```python
from build123d import *

# Parameters (mm, degrees)
SCHIZZO1_W                   = 22
SCHIZZO1_H                   = 10.6
ESTRUSIONE_ESTRUSIONE1_DEPTH = 15
TAGLIO_ESTRUSIONE3_REACH     = 23.409
SCHIZZO5_R                   = 1.75
SCHIZZO5_3_W                 = 6.5
SCHIZZO5_3_H                 = 30
TAGLIO_ESTRUSIONE4_DEPTH     = 0.6


with BuildPart() as part:
    # Schizzo1 → Estrusione-Estrusione1 (new, symmetric)
    with BuildSketch(Plane.XY):
        Rectangle(SCHIZZO1_W, SCHIZZO1_H)
    extrude(amount=ESTRUSIONE_ESTRUSIONE1_DEPTH, both=True)

    # Schizzo5 → Taglio-Estrusione3 (cut, up to next)
    with BuildSketch(Plane(origin=(0, 5.3, 0), x_dir=(1, 0, 0), z_dir=(0, 1, 0)), mode=Mode.PRIVATE) as taglio_estrusione3_sk1:
        with Locations(Location((6.5, 10.5, 0), (0, 0, 270))):
            Circle(SCHIZZO5_R)
    taglio_estrusione3_tool1 = extrude(taglio_estrusione3_sk1.sketch, amount=-TAGLIO_ESTRUSIONE3_REACH, mode=Mode.PRIVATE) & part.part
    # Schizzo5 → Taglio-Estrusione3 (cut, up to next)
    with BuildSketch(Plane(origin=(0, 5.3, 0), x_dir=(1, 0, 0), z_dir=(0, 1, 0)), mode=Mode.PRIVATE) as taglio_estrusione3_sk2:
        with Locations(Location((6.5, -10.5, 0), (0, 0, 270))):
            Circle(SCHIZZO5_R)
    taglio_estrusione3_tool2 = extrude(taglio_estrusione3_sk2.sketch, amount=-TAGLIO_ESTRUSIONE3_REACH, mode=Mode.PRIVATE) & part.part
    # Schizzo5 → Taglio-Estrusione3 (cut, up to next)
    with BuildSketch(Plane(origin=(0, 5.3, 0), x_dir=(1, 0, 0), z_dir=(0, 1, 0)), mode=Mode.PRIVATE) as taglio_estrusione3_sk3:
        with Locations(Location((-6.5, -10.5, 0), (0, 0, 270))):
            Circle(SCHIZZO5_R)
    taglio_estrusione3_tool3 = extrude(taglio_estrusione3_sk3.sketch, amount=-TAGLIO_ESTRUSIONE3_REACH, mode=Mode.PRIVATE) & part.part
    # Schizzo5 → Taglio-Estrusione3 (cut, up to next)
    with BuildSketch(Plane(origin=(0, 5.3, 0), x_dir=(1, 0, 0), z_dir=(0, 1, 0)), mode=Mode.PRIVATE) as taglio_estrusione3_sk4:
        with Locations(Location((-6.5, 10.5, 0), (0, 0, 270))):
            Circle(SCHIZZO5_R)
    taglio_estrusione3_tool4 = extrude(taglio_estrusione3_sk4.sketch, amount=-TAGLIO_ESTRUSIONE3_REACH, mode=Mode.PRIVATE) & part.part
    add(taglio_estrusione3_tool1.solids().sort_by_distance((6.5, 5.3, -10.5))[0], mode=Mode.SUBTRACT)
    add(taglio_estrusione3_tool2.solids().sort_by_distance((6.5, 5.3, 10.5))[0], mode=Mode.SUBTRACT)
    add(taglio_estrusione3_tool3.solids().sort_by_distance((-6.5, 5.3, 10.5))[0], mode=Mode.SUBTRACT)
    add(taglio_estrusione3_tool4.solids().sort_by_distance((-6.5, 5.3, -10.5))[0], mode=Mode.SUBTRACT)

    # Schizzo5_3 → Taglio-Estrusione4 (cut)
    with BuildSketch(Plane(origin=(0, 5.3, 0), x_dir=(1, 0, 0), z_dir=(0, 1, 0))):
        Rectangle(SCHIZZO5_3_W, SCHIZZO5_3_H)
    extrude(amount=-TAGLIO_ESTRUSIONE4_DEPTH, mode=Mode.SUBTRACT)


solid = part.part
```
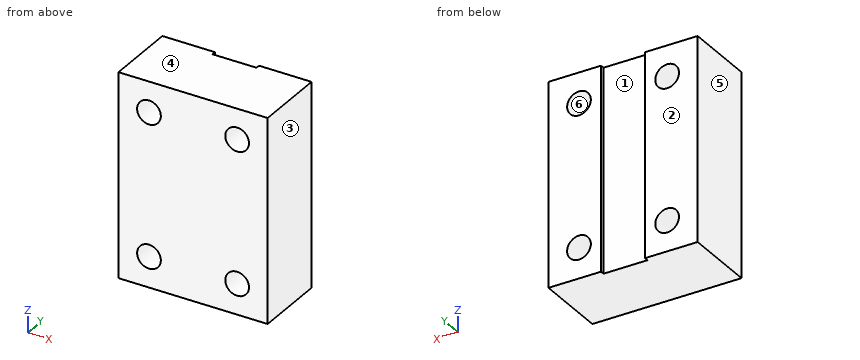
The model under review builds one solid part; all positions refer to its coordinate system, in mm. Face numbers are marked on the shaded views. A direction names the side the tool comes from. Round coordinates to 2 decimals unless told otherwise and drop trailing zeros. Loops run counter-clockwise (first coordinate to the right, second up) from the corner with the lowest first, then second, coordinate; pieces in that order, holes last. Notation, with made-up numbers: (14, 73.5) - (35, 73.5) arc R23 ccw to (35, 106.5) - close; hole circle Ø1 at (39, 53.5). An arc over 180 degrees is marked (long way). Use a Markdown table: item, result. Add a question column.
Q1. Insertion check: pin 1 Ø3 at (x, z) = (-6.5, -10.5) entering from -Y. The pin has a flat end and moves straight along its axis. Give the tip position at first contact, or say it passes through.
Q2. For probe 1 along X at (y, z) = (1, 10.5); probe 2 along Z at (x, y) = (-6.25, 2); probe 3 along X at (y, z) = (-4.25, -9), list the stretches that pass through material, from the lowest coordinate up.
Q3. Add section C-C (z = 10.5). State the section outline as (x, y) points.
Q4. Machinability: for the marked faces 1 and 2, which of the approach directions +Z, -Z, +X, -X, +Y, -Y give a long, thin tool a straight path to every point of the face, cutting with its end or side? Answer none if there is none.
Q5. Add section A-A (x = 6.5). State the section outline as (y, z) points.
Q6. Add section B-B (y = -1). State the section outline as (x, z) points.
Q7. Add section D-D (z = 3.25). State the section outline as (x, y) points.
Q8. The part is to be moulded in two halves that separate along X. For the marked faces 3, 4, 5 and 6, say which applies: pulls with the +X half, pulls with the -X half, needs draft (parallel to the pull), parting line crosses it, or undercut.
Worked answers:
| question | item | result |
|---|---|---|
| 1 | pin 1 | through |
| 2 | probe 1 | -11 to -8.25, -4.75 to 4.75, 8.25 to 11 |
| 2 | probe 2 | -15 to -12.23, -8.77 to 8.77, 12.23 to 15 |
| 2 | probe 3 | -11 to -7.4, -5.6 to 5.6, 7.4 to 11 |
| 3 | outline | (-11, -5.3) - (-8.25, -5.3) - (-8.25, 5.3) - (-11, 5.3) - close; (-4.75, -5.3) - (4.75, -5.3) - (4.75, 5.3) - (3.25, 5.3) - (3.25, 4.7) - (-3.25, 4.7) - (-3.25, 5.3) - (-4.75, 5.3) - close; (8.25, -5.3) - (11, -5.3) - (11, 5.3) - (8.25, 5.3) - close |
| 4 | face 1 | +Z, -Z, +Y |
| 4 | face 2 | +Z, -Z, +X, -X, +Y |
| 5 | outline | (-5.3, -15) - (5.3, -15) - (5.3, -12.25) - (-5.3, -12.25) - close; (-5.3, -8.75) - (5.3, -8.75) - (5.3, 8.75) - (-5.3, 8.75) - close; (-5.3, 12.25) - (5.3, 12.25) - (5.3, 15) - (-5.3, 15) - close |
| 6 | outline | (-11, -15) - (11, -15) - (11, 15) - (-11, 15) - close; hole circle Ø3.5 at (-6.5, -10.5); hole circle Ø3.5 at (-6.5, 10.5); hole circle Ø3.5 at (6.5, -10.5); hole circle Ø3.5 at (6.5, 10.5) |
| 7 | outline | (-11, -5.3) - (11, -5.3) - (11, 5.3) - (3.25, 5.3) - (3.25, 4.7) - (-3.25, 4.7) - (-3.25, 5.3) - (-11, 5.3) - close |
| 8 | face 3 | pulls with the +X half |
| 8 | face 4 | needs draft |
| 8 | face 5 | pulls with the -X half |
| 8 | face 6 | undercut |
